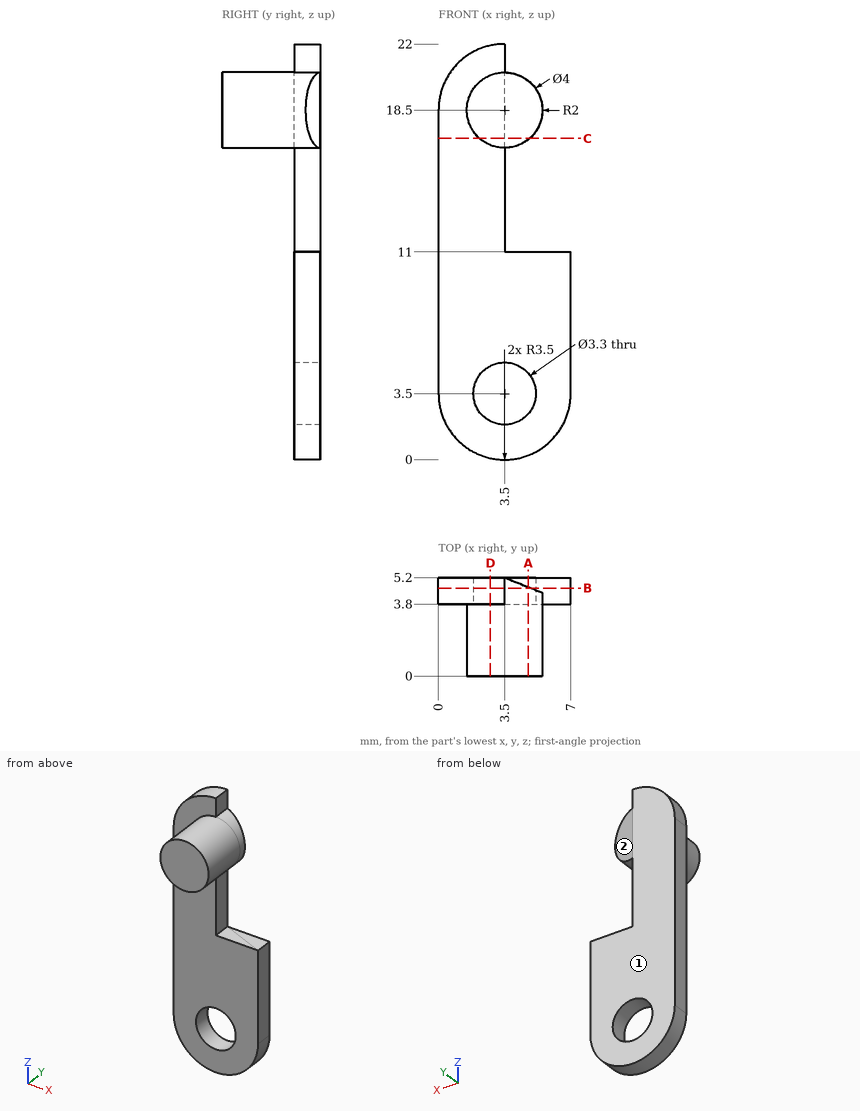
For this review, use the dimensioned drawing (mm, ordinates from the lowest corner) and the shaded views. A direction names the side the tool comes from. Give positions to 0.01 mm unless a question says otherwise; leave off trailing zeros. Order: outer loops, then holes, each group sorted by start corner. A loop starts at its lowest first (then second) coordinate and runs counter-clockwise, first axis right, second up. Notation, with made-up numbers: (71.25, 61.5) - (104.25, 61.5) arc R32 cw to (104.25, 94.5) - close; hole circle Ø10 at (13.25, 14.25). An arc over 180 degrees is marked (long way). Use a Markdown table: item, result. Add a question column.
(1) Add section C-C on z = 17. Give the boundary of the cut face in (x, y), then the cut area to 3 significant figures.
(2) Clearance check with flat-ended pins moving along their axes: P1, Ø4, axis at x = 3.5, z = 3.5, coming from the -Y side; P2, Ø0.7, axis at y = 4.5, z = 14.5, coming from the +X side; P3, Ø0.7, axis at x = 5, y = 4.5, coming from the +Z side. State where each tip first meets the part, or that it passes through.
(3) Add section D-D on x = 2.75. Give the boundary of the cut face in (y, z).
(4) Wall thickness on probe 1 along X at (y, z) = (4.65, 3.5); probe 2 along Z at (x, y) = (4.5, 4.5); probe 3 along Z at (x, y) = (4, 4.9): over which ranges is each line inside the solid? List them lowest first. Write a range as [from, to].
(5) Add section A-A on x = 4.75. Give the boundary of the cut face in (y, z).
(6) Add section B-B on y = 4.65. Give the boundary of the cut face in (x, z) (3 decimals), then the cut area to 3 significant figures.
(7) Machinability: for the marked faces 1 and 2, which of the approach directions +Z, -Z, +X, -X, +Y, -Y give a long, thin tool a straight path to every point of the face, cutting with its end or side? Answer none if there is none.
Report:
| question | item | result |
|---|---|---|
| 1 | outline | (0, 3.8) - (2.18, 3.8) - (2.18, 0) - (4.82, 0) - (4.82, 4.67) - (3.5, 5.2) - (0, 5.2) - close |
| 1 | area | 16.5 mm² |
| 2 | P1 | stops at y = 3.8 |
| 2 | P2 | stops at x = 3.5 |
| 2 | P3 | stops at z = 20.14 |
| 3 | outline | (0, 16.65) - (3.8, 16.65) - (3.8, 4.97) - (5.2, 4.97) - (5.2, 21.92) - (3.8, 21.92) - (3.8, 20.35) - (0, 20.35) - close; (3.8, 0.08) - (5.2, 0.08) - (5.2, 2.03) - (3.8, 2.03) - close |
| 4 | probe 1 | x = [0, 1.85], [5.15, 7] |
| 4 | probe 2 | z = [0.15, 2.19], [4.81, 11], [16.77, 20.23] |
| 4 | probe 3 | z = [0.04, 1.93], [5.07, 11], [16.56, 20.44] |
| 5 | outline | (0, 16.94) - (4.7, 16.94) - (4.7, 20.06) - (0, 20.06) - close; (3.8, 0.23) - (5.2, 0.23) - (5.2, 2.42) - (3.8, 2.42) - close; (3.8, 4.58) - (5.2, 4.58) - (5.2, 11) - (3.8, 11) - close |
| 6 | outline | (0, 3.5) arc R3.5 ccw to (7, 3.5) - (7, 11) - (3.5, 11) - (3.5, 16.5) arc R2 ccw to (4.875, 17.048) - (4.875, 19.952) arc R2 ccw to (3.5, 20.5) - (3.5, 22) arc R3.5 ccw to (0, 18.5) - close; hole circle Ø3.3 at (3.5, 3.5) |
| 6 | area | 104 mm² |
| 7 | face 1 | +Z, -Z, +X, -X, +Y |
| 7 | face 2 | +Z, +X, +Y |
